Input: part model. Units: mm. Frame: model coordinates. A direction names the side the tool comes from. Round coordinates to 2 decimals unless told otherwise and drop trailing zeros. Loops run counter-clockwise (first coordinate to the right, second up) from the corner with the lowest first, then second, coordinate; pieces in that order, holes last. Notation, with made-up numbers: (61, 54.5) -> (112, 54.5) arc R16 ccw to (112, 65.5) -> close; hole circle Ø11 at (86.5, 49). An arc over 180 degrees is marked (long way). Answer as a JSON object with one key per item and string values. Group by question number.
Item 1: Section query B-B on x = -445.5. Return loops of the section in (y, z) (3 decimals), and give its area (3 significant figures).
Item 2: Set-up query: faces 5 (the flat face through (-445, -49, 0)), 6 (the flat face through (-467.777, -91, 2)). Return all of +Z, -Z, +X, -X, +Y, -Y with unobstructed straight access to the full face (end or side cutting, diameter ignored); none if empty.
Item 3: Material intervals for line 1 (Y direction, x = -465.5, z = 2.85); line 2 (Y direction, x = -401.5, z = 1.4); line 3 (X direction, y = -60, z = 0.7), sorted ascending. Write a range as [from, to].
Item 4: Section query A-A on y = -94. Return loops of the section in (x, z) (3 decimals), and give its area (3 significant figures).
Item 5: Section query C-C on x = -473.5. Return loops of the section in (y, z) (3 decimals), and give its area (3 significant figures).
Item 6: Section query D-D on z = 0.8. Count the separate pieces of the cut face and the enclosed holes in it, and give its area (3 significant figures).
Item 7: Draft query along Y for faces 1 (the flat face through (-504.29, -50, 2)), 2 (the flat face through (-419.517, -33, 2)), 3 (the cylindrical face through (-500.668, -116.459, 1.565)), 4 (the cylindrical face through (-391.347, -0.81, 1.565)). Return one class per face: released by +Y, released by -Y, zero draft, split by the parting line, or undercut.
from build123d import *

# Parameters (mm, degrees)
F0_R     = 1.9939
F0_R_2   = 1.524
F0_W     = 48.26
F0_H     = 15.391365
F0_H_2   = 14.904542
F1_DEPTH = 3.175


with BuildPart() as f1:
    # F0 (on Top) → F1 (new body)
    with BuildSketch(Plane.XY):
        with BuildLine():
            Line((-395.704613, 19.42213), (-491.589613, 19.42213))
            ThreePointArc((-491.589613, 19.42213), (-500.569869, 15.702386), (-504.289613, 6.72213))
            Line((-504.289613, 6.72213), (-504.289613, -107.57787))
            ThreePointArc((-504.289613, -107.57787), (-500.569869, -116.558126), (-491.589613, -120.27787))
            Line((-491.589613, -120.27787), (-396.339613, -120.27787))
            ThreePointArc((-396.339613, -120.27787), (-387.359356, -116.558126), (-383.639613, -107.57787))
            Line((-383.639613, -107.57787), (-383.639613, 7.35713))
            ThreePointArc((-383.639613, 7.35713), (-387.173369, 15.888373), (-395.704613, 19.42213))
        make_face()
        with Locations((-497.939613, -112.65787)):
            Circle(F0_R, mode=Mode.SUBTRACT)
        with Locations((-485.874613, -112.65787)):
            Circle(F0_R, mode=Mode.SUBTRACT)
        with Locations((-497.939613, -98.68787)):
            Circle(F0_R, mode=Mode.SUBTRACT)
        with Locations((-473.809613, -112.65787)):
            Circle(F0_R, mode=Mode.SUBTRACT)
        with Locations((-461.744613, -112.65787)):
            Circle(F0_R, mode=Mode.SUBTRACT)
        with Locations((-449.679613, -112.65787)):
            Circle(F0_R, mode=Mode.SUBTRACT)
        with Locations((-497.939613, -84.71787)):
            Circle(F0_R, mode=Mode.SUBTRACT)
        with Locations((-497.939613, -70.74787)):
            Circle(F0_R, mode=Mode.SUBTRACT)
        with Locations((-497.939613, -56.77787)):
            Circle(F0_R, mode=Mode.SUBTRACT)
        with Locations((-462.697113, -60.680724)):
            Circle(F0_R_2, mode=Mode.SUBTRACT)
        with Locations((-437.614613, -112.65787)):
            Circle(F0_R, mode=Mode.SUBTRACT)
        with Locations((-425.549613, -112.65787)):
            Circle(F0_R, mode=Mode.SUBTRACT)
        with Locations((-443.647113, -90.65491)):
            Rectangle(F0_W, F0_H, mode=Mode.SUBTRACT)
        with Locations((-413.484613, -112.65787)):
            Circle(F0_R, mode=Mode.SUBTRACT)
        with Locations((-401.419613, -112.65787)):
            Circle(F0_R, mode=Mode.SUBTRACT)
        with Locations((-389.354613, -112.65787)):
            Circle(F0_R, mode=Mode.SUBTRACT)
        with Locations((-389.354613, -98.68787)):
            Circle(F0_R, mode=Mode.SUBTRACT)
        with Locations((-434.757113, -60.680724)):
            Circle(F0_R_2, mode=Mode.SUBTRACT)
        with Locations((-389.354613, -84.71787)):
            Circle(F0_R, mode=Mode.SUBTRACT)
        with Locations((-389.354613, -70.74787)):
            Circle(F0_R, mode=Mode.SUBTRACT)
        with Locations((-389.354613, -56.77787)):
            Circle(F0_R, mode=Mode.SUBTRACT)
        with Locations((-497.939613, -42.80787)):
            Circle(F0_R, mode=Mode.SUBTRACT)
        with Locations((-497.939613, -28.83787)):
            Circle(F0_R, mode=Mode.SUBTRACT)
        with Locations((-497.939613, -14.86787)):
            Circle(F0_R, mode=Mode.SUBTRACT)
        with Locations((-497.939613, -0.89787)):
            Circle(F0_R, mode=Mode.SUBTRACT)
        with Locations((-497.939613, 13.07213)):
            Circle(F0_R, mode=Mode.SUBTRACT)
        with Locations((-485.874613, 13.07213)):
            Circle(F0_R, mode=Mode.SUBTRACT)
        with Locations((-467.777113, -9.880724)):
            Circle(F0_R_2, mode=Mode.SUBTRACT)
        with Locations((-473.809613, 13.07213)):
            Circle(F0_R, mode=Mode.SUBTRACT)
        with Locations((-461.744613, 13.07213)):
            Circle(F0_R, mode=Mode.SUBTRACT)
        with Locations((-449.679613, 13.07213)):
            Circle(F0_R, mode=Mode.SUBTRACT)
        with Locations((-443.647113, -33.013412)):
            Rectangle(F0_W, F0_H_2, mode=Mode.SUBTRACT)
        with Locations((-389.354613, -42.80787)):
            Circle(F0_R, mode=Mode.SUBTRACT)
        with Locations((-389.354613, -28.83787)):
            Circle(F0_R, mode=Mode.SUBTRACT)
        with Locations((-419.517113, -9.880724)):
            Circle(F0_R_2, mode=Mode.SUBTRACT)
        with Locations((-437.614613, 13.07213)):
            Circle(F0_R, mode=Mode.SUBTRACT)
        with Locations((-425.549613, 13.07213)):
            Circle(F0_R, mode=Mode.SUBTRACT)
        with Locations((-389.354613, -14.86787)):
            Circle(F0_R, mode=Mode.SUBTRACT)
        with Locations((-389.354613, -0.89787)):
            Circle(F0_R, mode=Mode.SUBTRACT)
        with Locations((-413.484613, 13.07213)):
            Circle(F0_R, mode=Mode.SUBTRACT)
        with Locations((-401.419613, 13.07213)):
            Circle(F0_R, mode=Mode.SUBTRACT)
        with Locations((-389.354613, 13.07213)):
            Circle(F0_R, mode=Mode.SUBTRACT)
    extrude(amount=F1_DEPTH)


solid = f1.part
Solved:
{
 "1": {"outline": "(-120.278, 0) -> (-98.351, 0) -> (-98.351, 3.175) -> (-120.278, 3.175) -> close; (-82.959, 0) -> (-40.466, 0) -> (-40.466, 3.175) -> (-82.959, 3.175) -> close; (-25.561, 0) -> (19.422, 0) -> (19.422, 3.175) -> (-25.561, 3.175) -> close", "area": "347 mm²"},
 "2": {"face 5": "-Z, +X, -X, +Y, -Y", "face 6": "+Z, -Z"},
 "3": {"line 1": "[-120.28, -98.35], [-82.96, -40.47], [-25.56, 19.42]", "line 2": "[-120.28, -114.65], [-110.67, 11.08], [15.06, 19.42]", "line 3": "[-504.29, -464.06], [-461.33, -436.12], [-433.39, -383.64]"},
 "4": {"outline": "(-504.29, 0) -> (-467.777, 0) -> (-467.777, 3.175) -> (-504.29, 3.175) -> close; (-419.517, 0) -> (-383.64, 0) -> (-383.64, 3.175) -> (-419.517, 3.175) -> close", "area": "230 mm²"},
 "5": {"outline": "(-120.278, 0) -> (-114.628, 0) -> (-114.628, 3.175) -> (-120.278, 3.175) -> close; (-110.688, 0) -> (11.102, 0) -> (11.102, 3.175) -> (-110.688, 3.175) -> close; (15.042, 0) -> (19.422, 0) -> (19.422, 3.175) -> (15.042, 3.175) -> close", "area": "419 mm²"},
 "6": {"separate pieces": "1", "enclosed holes": "42", "area": "14,800 mm²"},
 "7": {"face 1": "zero draft", "face 2": "undercut", "face 3": "released by -Y", "face 4": "undercut"}
}
